```python
from build123d import *

# Parameters (mm, degrees)
BOSS_EXTRUDE1_DEPTH       = 5
F_8_CLEARANCE_HOLE1_D     = 4.4958
F_8_CLEARANCE_HOLE1_DEPTH = 17
F_8_CLEARANCE_HOLE1_TIP   = 1.350674586
SKETCH3_W                 = 3
SKETCH3_H                 = 6
BOSS_EXTRUDE2_DEPTH       = 18
RIB2_REACH                = 59.744
SKETCH17_WALL_W           = 124.92066757
SKETCH17_WALL_H           = 6
RIB3_REACH                = 59.054
SKETCH18_WALL_W           = 123.798893364
SKETCH18_WALL_H           = 6
F_8_CLEARANCE_HOLE2_D     = 4.4958
F_8_CLEARANCE_HOLE2_DEPTH = 17
F_8_CLEARANCE_HOLE2_TIP   = 1.350674586


with BuildPart() as part:
    # Sketch1 → Boss-Extrude1 (new body)
    with BuildSketch(Plane(origin=(0, 0, 0), x_dir=(1, 0, 0), z_dir=(0, 1, 0))):
        Polygon((-14.338976611, 0), (30.661023389, 0), (8.161023389, 55.621488653), align=None)
    extrude(amount=BOSS_EXTRUDE1_DEPTH)

    # #8 Clearance Hole1
    with Locations(Plane(origin=(22.377803879, 0, -3.25), x_dir=(0, 0, -1), z_dir=(0, -1, 0))):
        with Locations((0, 0), (0, -27.25), (30.001031232, -13.625)):
            Hole(F_8_CLEARANCE_HOLE1_D / 2, depth=F_8_CLEARANCE_HOLE1_DEPTH)
            with Locations((0, 0, -(F_8_CLEARANCE_HOLE1_DEPTH + F_8_CLEARANCE_HOLE1_TIP / 2))):  # 118° drill point
                Cone(0, F_8_CLEARANCE_HOLE1_D / 2, F_8_CLEARANCE_HOLE1_TIP, mode=Mode.SUBTRACT)

    # Sketch3 → Boss-Extrude2 (add)
    with BuildSketch(Plane(origin=(0, 0, 0), x_dir=(-1, 0, 0), z_dir=(0, -1, 0))):
        with Locations((-9.161023389, 42.5)):
            Rectangle(SKETCH3_W, SKETCH3_H)
        with Locations((-9.161023389, 8)):
            Rectangle(SKETCH3_W, SKETCH3_H)
    extrude(amount=BOSS_EXTRUDE2_DEPTH)

    # Sketch17 wall → Rib2 (add, up to next)
    with BuildSketch(Plane(origin=(6.411023389, -3.5, -45.5), x_dir=(-0.336336396998, 0.941741911595, 0), z_dir=(0.941741911595, 0.336336396998, 0)), mode=Mode.PRIVATE) as rib2_sk1:
        with Locations((0, 3)):
            Rectangle(SKETCH17_WALL_W, SKETCH17_WALL_H)
    rib2_tool1 = extrude(rib2_sk1.sketch, amount=RIB2_REACH, mode=Mode.PRIVATE) - part.part
    add(rib2_tool1.solids().sort_by_distance((6.411023389, -3.5, -45.5))[0])

    # Sketch18 wall → Rib3 (add, up to next)
    with BuildSketch(Plane(origin=(6.411023389, -3.36354082, -11), x_dir=(-0.32507212999, 0.945689225012, 0), z_dir=(0.945689225012, 0.32507212999, 0)), mode=Mode.PRIVATE) as rib3_sk1:
        with Locations((0, 3)):
            Rectangle(SKETCH18_WALL_W, SKETCH18_WALL_H)
    rib3_tool1 = extrude(rib3_sk1.sketch, amount=RIB3_REACH, mode=Mode.PRIVATE) - part.part
    add(rib3_tool1.solids().sort_by_distance((6.411023389, -3.36354082, -11))[0])

    # #8 Clearance Hole2
    with Locations(Plane(origin=(7.661023389, -14, -42.5), x_dir=(0, 0, -1), z_dir=(-1, 0, 0))):
        with Locations((0, 0), (-34.5, 0)):
            Hole(F_8_CLEARANCE_HOLE2_D / 2, depth=F_8_CLEARANCE_HOLE2_DEPTH)
            with Locations((0, 0, -(F_8_CLEARANCE_HOLE2_DEPTH + F_8_CLEARANCE_HOLE2_TIP / 2))):  # 118° drill point
                Cone(0, F_8_CLEARANCE_HOLE2_D / 2, F_8_CLEARANCE_HOLE2_TIP, mode=Mode.SUBTRACT)


solid = part.part
```
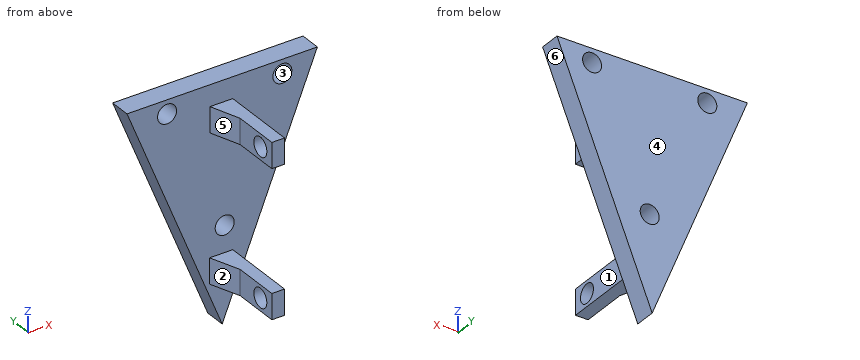
The model under review builds one solid part; all positions refer to its coordinate system, in mm. Face numbers are marked on the shaded views. A direction names the side the tool comes from. Round coordinates to 2 decimals unless told otherwise and drop trailing zeros. Write each loop counter-clockwise with the first axis right and the second up, starting at its lowest first coordinate (ties: lowest second). Pieces come first, ordered by that corner, then holes.
(1) Machinability: for the marked faces 1 and 2, which of the approach directions +Z, -Z, +X, -X, +Y, -Y give a long, thin tool a straight path to every point of the face, cutting with its end or side? Answer none if there is none.
(2) We need section D-D on z = -3.25. Give the boundary of the cut face in (x, y), and give its area (3 significant figures).
(3) We need section A-A on y = -14. Give the boundary of the cut face in (x, z), and give its area (3 significant figures).
(4) Wall thickness on L1, parallel to Z at x = 9.6, y = -14; L2, parallel to X at y = 2.7, z = -3.25; L3, parallel to Y at x = 8.6, z = -8: over which ranges is each line inside the solid? List them lowest first.
(5) We need section C-C on y = -5. Give the boundary of the cut face in (x, z).
(6) Insertion check: pin 1 (5 mm diameter, centred on y = -14, z = -8, fed in from -X); pin 2 (2 mm diameter, centred on x = 23, z = -6, fed in from -Y); pin 3 (6.5 mm diameter, centred on y = -13, z = -41, fed in from +X). Each pin has a flat end and moves straight along its axis. Give the tip position at first contact, or say it passes through.
(7) Mouldability with a two-part tool opening along X and no side actions: class the marked faces 3, 4, 5 and 6 as +X half, -X half, draft (parallel to the pull), parting line (faces both ways), or undercut.
(8) We need section B-B on z = -42.5. Give the boundary of the cut face in (x, y), and give its area (3 significant figures).
Findings below:
1. face 1: +Z, -Z, +X, -Y
1. face 2: +Z, -Z, -X, -Y
2. outline: (-13.02, 0) - (-7.12, 0) - (-7.12, 5) - (-13.02, 5) - close; (-2.62, 0) - (20.13, 0) - (20.13, 5) - (-2.62, 5) - close; (24.63, 0) - (29.35, 0) - (29.35, 5) - (24.63, 5) - close
2. area: 167 mm2
3. outline: (7.66, -45.5) - (10.66, -45.5) - (10.66, -44.75) - (7.66, -44.75) - close; (7.66, -40.25) - (10.66, -40.25) - (10.66, -39.5) - (7.66, -39.5) - close; (7.66, -11) - (10.66, -11) - (10.66, -10.25) - (7.66, -10.25) - close; (7.66, -5.75) - (10.66, -5.75) - (10.66, -5) - (7.66, -5) - close
3. area: 9.03 mm2
4. L1: z = -45.5 to -44.75, -40.25 to -39.5, -11 to -10.25, -5.75 to -5
4. L2: x = -13.02 to -7.12, -2.62 to 20.13, 24.63 to 29.35
4. L3: y = -18 to -16.25, -11.75 to 5
5. outline: (6.95, -45.5) - (10.66, -45.5) - (10.66, -39.5) - (6.95, -39.5) - close; (6.97, -11) - (10.66, -11) - (10.66, -5) - (6.97, -5) - close
6. pin 1: stops at x = 7.66
6. pin 2: stops at y = 0
6. pin 3: stops at x = 10.66
7. face 3: undercut
7. face 4: draft
7. face 5: -X half
7. face 6: +X half
8. outline: (2.85, 0) - (5.16, 0) - (7.66, -7) - (7.66, -11.75) - (10.66, -11.75) - (10.66, 0) - (13.47, 0) - (13.47, 5) - (2.85, 5) - close; (7.66, -18) - (10.66, -18) - (10.66, -16.25) - (7.66, -16.25) - close
8. area: 102 mm2
